Input: dimensioned drawing with shaded views. Units: mm. Origin: part minimum x, y, z. A direction names the side the tool comes from. Coordinates: 2 decimals unless noted, no trailing zeros. Order: outer loops, then holes, each group sorted by start corner. A loop starts at its lowest first (then second) coordinate and runs counter-clockwise, first axis right, second up. Notation, with made-up numbers: (-18, 83) -> (-9, 83) arc R31 ccw to (-9, 122) -> close; hole circle Ø5 at (-7, 75). An arc over 180 degrees is marked (long way). Write item = value, one per line. Start each with the question number.
Item 1: Set-up query: the marked faces 1 and 2. Return all of +Z, -Z, +X, -X, +Y, -Y with unobstructed straight access to the full face (end or side cutting, diameter ignored); none if empty.
Item 2: Section query A-A (x = 107). Output: boundary loops of the cut face in (y, z).
Item 3: Mould query, pull axis X, two halves, no side actions, for the marked faces 3, 4 and 5. Classes: released by +X, released by -X, zero draft, split by the parting line, or undercut.
Item 4: Section query C-C (x = 83). Output: boundary loops of the cut face in (y, z).
Item 5: Ray query, line 1 along Z through (x, y) = (107, 180); line 2 along X through (y, z) = (180, 100); line 3 along Y through (x, z) = (66, 110.5). Return the intervals inside material, ascending. Write a range as [from, to].
Item 6: Section query D-D (z = 247.55). Output: boundary loops of the cut face in (x, y) (1 decimal).
Item 7: Section query B-B (z = 100). Output: boundary loops of the cut face in (x, y).
Item 8: Contact query for flat-ended pins moving along their axis: pin 1 (8 mm diameter, centred on y = 15.5, z = 226.5, fed in from -X); pin 2 (10 mm diameter, centred on x = 145.5, y = 42, fed in from +Z); pin 3 (5 mm diameter, centred on x = 89, y = 150, fed in from -Z). Output: stop coordinate, or through.
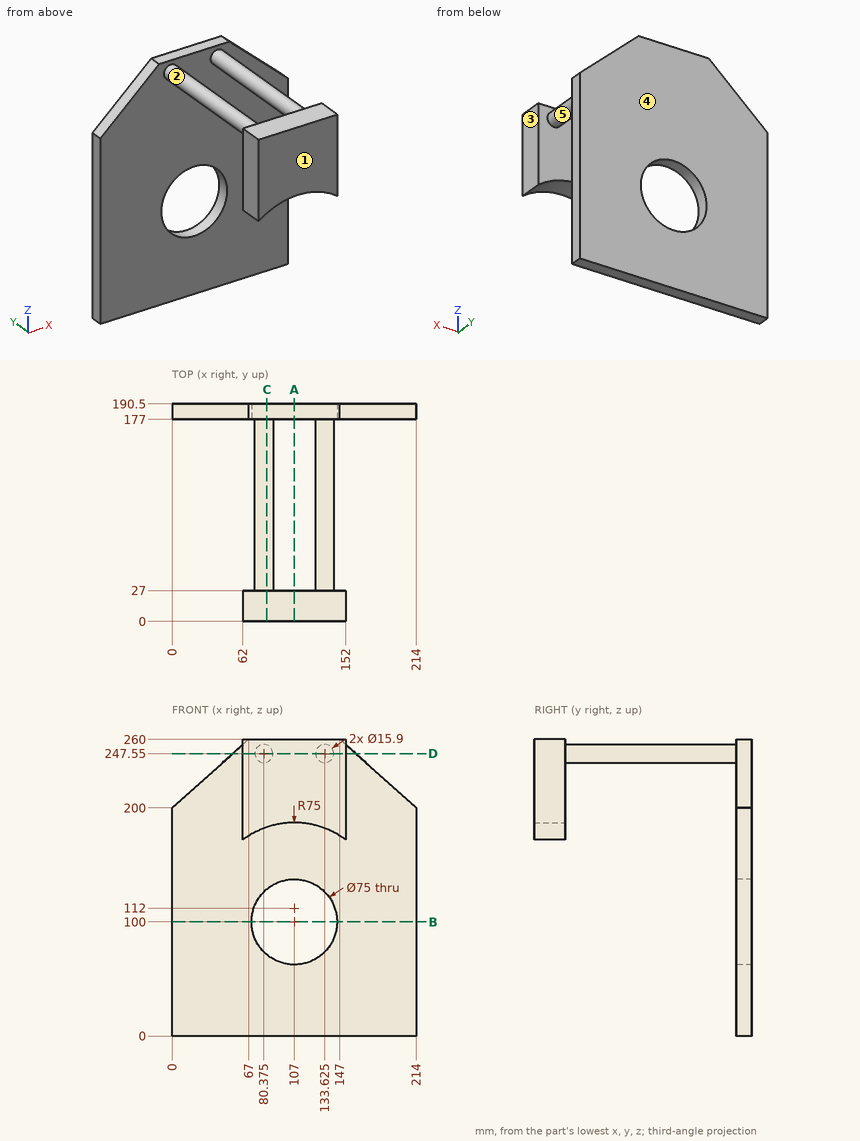
Computed:
q1.face_1 = +Z, -Z, +X, -X, -Y
q1.face_2 = none
q2.outline = (0, 187) -> (27, 187) -> (27, 260) -> (0, 260) -> close; (177, 0) -> (190.5, 0) -> (190.5, 62.5) -> (177, 62.5) -> close; (177, 137.5) -> (190.5, 137.5) -> (190.5, 260) -> (177, 260) -> close
q3.face_3 = released by +X
q3.face_4 = zero draft
q3.face_5 = undercut
q4.outline = (0, 183.06) -> (27, 183.06) -> (27, 240.05) -> (177, 240.05) -> (177, 128.81) -> (190.5, 128.81) -> (190.5, 260) -> (177, 260) -> (177, 255.05) -> (27, 255.05) -> (27, 260) -> (0, 260) -> close; (177, 0) -> (190.5, 0) -> (190.5, 71.19) -> (177, 71.19) -> close
q5.line_1 = [0, 62.5], [137.5, 260]
q5.line_2 = [0, 69.5], [144.5, 214]
q5.line_3 = [177, 190.5]
q6.outline = (53.1, 177) -> (72.4, 177) -> (72.4, 27) -> (62, 27) -> (62, 0) -> (152, 0) -> (152, 27) -> (141.6, 27) -> (141.6, 177) -> (160.9, 177) -> (160.9, 190.5) -> (53.1, 190.5) -> close; hole (88.3, 27) -> (125.7, 27) -> (125.7, 177) -> (88.3, 177) -> close
q7.outline = (0, 177) -> (69.5, 177) -> (69.5, 190.5) -> (0, 190.5) -> close; (144.5, 177) -> (214, 177) -> (214, 190.5) -> (144.5, 190.5) -> close
q8.pin_1 = 62
q8.pin_2 = 251.54
q8.pin_3 = 242.48
